from build123d import *

# Parameters (mm, degrees)
SKETCH1_W               = 200
SKETCH1_H               = 70
BOSS_EXTRUDE1_DEPTH     = 55
SKETCH3_W               = 50
SKETCH3_H               = 55
CUT_EXTRUDE1_DEPTH      = 23
CUT_EXTRUDE2_DEPTH      = 134.88427839
CUT_EXTRUDE2_DEPTH_BACK = 134.88427839
SKETCH4_OUTSIDE_W       = 245.784
SKETCH4_OUTSIDE_H       = 100.784
FILLET2_R               = 2
CUT_EXTRUDE6_DEPTH      = 133.153320217
CUT_EXTRUDE6_DEPTH_BACK = 133.153320217
SKETCH11_R              = 2.5
SKETCH12_W              = 106.420184481
SKETCH12_H              = 81.22852992
CUT_EXTRUDE7_DEPTH      = 25
CUT_EXTRUDE8_DEPTH      = 127.208161551
CUT_EXTRUDE9_DEPTH      = 50
SKETCH15_R              = 2.5
SKETCH15_R_2            = 1.5
CUT_EXTRUDE10_DEPTH     = 50
SKETCH16_W              = 5
SKETCH16_H              = 10
CUT_EXTRUDE11_DEPTH     = 162.677147573


with BuildPart() as part:
    # Sketch1 → Boss-Extrude1 (new body)
    with BuildSketch(Plane(origin=(0, 0, 0), x_dir=(1, 0, 0), z_dir=(0, 1, 0))):
        Rectangle(SKETCH1_W, SKETCH1_H)
    extrude(amount=BOSS_EXTRUDE1_DEPTH)

    # Sketch3 → Cut-Extrude1 (cut, symmetric)
    with BuildSketch(Plane.XY):
        with Locations((75, 27.5)):
            Rectangle(SKETCH3_W, SKETCH3_H)
    extrude(amount=CUT_EXTRUDE1_DEPTH, both=True, mode=Mode.SUBTRACT)

    # Sketch4 outside → Cut-Extrude2 (cut, two sides: drawn at the far end of the back side and taken through both)
    with BuildSketch(Plane.XY.offset(35).offset(-CUT_EXTRUDE2_DEPTH_BACK)):
        with Locations((0, 27.5)):
            Rectangle(SKETCH4_OUTSIDE_W, SKETCH4_OUTSIDE_H)
        with BuildLine():
            ThreePointArc((-72.5, 53.5), (-98.5, 27.5), (-72.5, 1.5))
            ThreePointArc((-72.5, 1.5), (2.267755531, 6.809398073), (77.063073628, 1.90354792))
            ThreePointArc((77.063073628, 1.90354792), (98.5, 27.5), (77.063073628, 53.09645208))
            ThreePointArc((77.063073628, 53.09645208), (2.267755531, 48.190601927), (-72.5, 53.5))
        make_face(mode=Mode.SUBTRACT)
    extrude(amount=CUT_EXTRUDE2_DEPTH + CUT_EXTRUDE2_DEPTH_BACK, mode=Mode.SUBTRACT)

    # Fillet2
    fillet2_edges = [part.edges().sort_by_distance(p)[0] for p in [
        (2.267755531, 48.190601927, -35),
        (2.267755531, 6.809398073, -35),
        (2.267755531, 48.190601927, 35),
        (2.267755531, 6.809398073, 35),
    ]]
    fillet(fillet2_edges, radius=FILLET2_R)

    # Sketch11 → Cut-Extrude6 (cut, two sides: drawn at the far end of the back side and taken through both)
    with BuildSketch(Plane.XY.offset(35).offset(-CUT_EXTRUDE6_DEPTH_BACK)):
        with Locations((-76.15, 27.5)):
            Circle(SKETCH11_R)
    extrude(amount=CUT_EXTRUDE6_DEPTH + CUT_EXTRUDE6_DEPTH_BACK, mode=Mode.SUBTRACT)

    # Sketch12 → Cut-Extrude7 (cut, symmetric)
    with BuildSketch(Plane.XY):
        with Locations((-91.710092241, 25.80773896)):
            Rectangle(SKETCH12_W, SKETCH12_H)
    extrude(amount=CUT_EXTRUDE7_DEPTH, both=True, mode=Mode.SUBTRACT)

    # Sketch13 → Cut-Extrude8 (cut, through all)
    with BuildSketch(Plane(origin=(0, 0, 23), x_dir=(-1, 0, 0), z_dir=(0, 0, -1))):
        with BuildLine():
            Line((-50, 4.863495472), (-50, 50.136504528))
            ThreePointArc((-50, 50.136504528), (-63.549853932, 51.449003205), (-77.063073628, 53.09645208))
            ThreePointArc((-77.063073628, 53.09645208), (-98.5, 27.5), (-77.063073628, 1.90354792))
            ThreePointArc((-77.063073628, 1.90354792), (-63.549853932, 3.550996795), (-50, 4.863495472))
        make_face()
    extrude(amount=-CUT_EXTRUDE8_DEPTH, mode=Mode.SUBTRACT)

    # Sketch14 → Cut-Extrude9 (cut)
    with BuildSketch(Plane.XY.offset(-23)):
        Polygon((50, 4.863495472), (79.442513565, -11.304195271), (157.593662914, 0), (128.462884047, 83.234297684), (50, 50.136504528), (98.5, 50.136504528), (98.5, 4.863495472), align=None)
    extrude(amount=-CUT_EXTRUDE9_DEPTH, mode=Mode.SUBTRACT)

    # Sketch15 → Cut-Extrude10 (cut)
    with BuildSketch(Plane.XY.offset(-23)):
        with Locations((71.15, 27.5)):
            Circle(SKETCH15_R)
        with Locations((55.650219356, 42.999780644)):
            Circle(SKETCH15_R_2)
        with Locations((86.649780644, 42.999780644)):
            Circle(SKETCH15_R_2)
        with Locations((86.649780644, 12.000219356)):
            Circle(SKETCH15_R_2)
        with Locations((55.650219356, 12.000219356)):
            Circle(SKETCH15_R_2)
    extrude(amount=-CUT_EXTRUDE10_DEPTH, mode=Mode.SUBTRACT)

    # Sketch16 → Cut-Extrude11 (cut, through all)
    with BuildSketch(Plane(origin=(50, 0, 0), x_dir=(0, 0, -1), z_dir=(1, 0, 0))):
        with Locations((20.5, 27.5)):
            Rectangle(SKETCH16_W, SKETCH16_H)
    extrude(amount=-CUT_EXTRUDE11_DEPTH, mode=Mode.SUBTRACT)


solid = part.part
CAD build for the part. Positions are in the model's coordinates, mm. A direction names the side the tool comes from. Coordinates: 2 decimals unless noted, no trailing zeros. Loops run counter-clockwise (first coordinate to the right, second up) from the corner with the lowest first, then second, coordinate; pieces in that order, holes last. Notation, with made-up numbers: (-30.5, 69.5) - (-11.5, 69.5) arc R25 ccw to (-11.5, 84.5) - close; hole circle Ø9 at (73, 50). An arc over 180 degrees is marked (long way). Use one line per item in the form item = value. Start each with the question number.
1) Band-saw the part on B-B (z = 31). Give the cut face in (x, y), and give its area (3 significant figures).
2) Band-saw the part on D-D (z = 12). Give the cut face in (x, y).
3) Tool access for faces 4 (the face through (-38.5, 27, 0)), 5 (the face through (6, 22.5, -20)), 6 (the face through (44, 28, -23)): list every direction of +Z, -Z, +X, -X, +Y, -Y with a clear straight run to the whole face (end or side of a thin tool).
4) Band-saw the part on A-A (y = 27.5). Give the cut face in (x, z), and give its area (3 significant figures).
5) Drill centre lines: L1, parallel to Y at x = 71.15, z = -30; L2, parallel to Z at x = -69.5, y = 39; L3, parallel to Z at x = 37.5, y = 31.5. Where is each one in solid material? Low to high. Write a range as from..to.
6) Flat gauge pins, fed straight in: pin 1 (6 mm diameter, centred on x = 56, y = 33.5, fed in from +Z); pin 2 (6 mm diameter, centred on y = 39.5, z = 7, fed in from +X); pin 3 (9.5 mm diameter, centred on x = 67, z = -26, fed in from +Y). Where does each tip first touch, or does it go through?
7) Two-plate mould, pull along X, no slides. Class faces 1 (the face through (1.439, 6.807, -0.462)), 2 (the face through (-98.494, 28.072, -30.07)), 3 (the face through (67, 50.137, -29)): +X half, -X half, draft (parallel to the pull), parting line (faces both ways), or undercut.
8) Band-saw the part on C-C (x = -76.15). State how many separate pieces and enclosed holes the cut face has, and give its area (3 significant figures).
Check values:
q1.outline = (-72.5, 1.5) arc R550 cw to (50, 4.86) - (50, 50.14) arc R550 cw to (-72.5, 53.5) arc R26 ccw to start; hole circle Ø5 at (-76.15, 27.5)
q1.area = 6,440 mm2
q2.outline = (-38.5, 5.19) arc R550 cw to (50, 4.86) - (50, 50.14) arc R550 cw to (-38.5, 49.81) - close
q3.face_4 = -X, +Y, -Y
q3.face_5 = +X, -X
q3.face_6 = +X
q4.outline = (-98.5, -35) - (-78.65, -35) - (-78.65, -25) - (-98.5, -25) - close; (-98.5, 25) - (-78.65, 25) - (-78.65, 35) - (-98.5, 35) - close; (-73.65, -35) - (68.65, -35) - (68.65, -23) - (-38.5, -23) - (-38.5, -25) - (-73.65, -25) - close; (-73.65, 25) - (-38.5, 25) - (-38.5, -18) - (50, -18) - (50, 35) - (-73.65, 35) - close; (73.65, -35) - (98.5, -35) - (98.5, -23) - (73.65, -23) - close
q4.area = 7,370 mm2
q5.L1 = 4.86..25, 30..50.14
q5.L2 = -35..-25, 25..35
q5.L3 = -35..-23, -18..35
q6.pin_1 = -23
q6.pin_2 = 50
q6.pin_3 = 50.14
q7.face_1 = undercut
q7.face_2 = -X half
q7.face_3 = draft
q8.separate_pieces = 4
q8.enclosed_holes = 0
q8.area = 929 mm2
